```python
from build123d import *

# Parameters (mm, degrees)
F0_W           = 40
F0_H           = 40
F0_R           = 0.75
F0_W_2         = 13
F0_H_2         = 14
F1_DEPTH       = 10
F3_DEPTH       = 7
F5_DEPTH       = 7
F6_W           = 1
F6_H           = 10
F7_DEPTH       = 3
F9_W           = 40
F9_H           = 40
F9_W_2         = 13
F9_H_2         = 14
F10_DEPTH      = 5
F8_W           = 16.9138771733
F8_H           = 9.9888166223
F11_DEPTH      = 5
F13_W          = 3
F13_H          = 1.8063458446
F13_H_2        = 1.6774383839
F14_DEPTH      = 7
F15_W          = 50
F15_H          = 50
F15_W_2        = 40
F15_H_2        = 40
F16_DEPTH      = 10
F16_DEPTH_BACK = 5
F8_W_2         = 1
F8_W_3         = 4.5249774149
F8_W_4         = 11.3888997585
F18_DEPTH      = 5
F17_R          = 2.5
F19_DEPTH      = 15
F20_W          = 1
F20_H          = 18
F20_W_2        = 1.1054268107
F20_H_2        = 4.0429783403
F20_H_3        = 1.6282203142
F20_W_3        = 3.4427661449
F20_H_4        = 4.0144510567
F21_DEPTH      = 7
F22_W          = 1.9634229802
F22_H          = 1
F23_DEPTH      = 3


with BuildPart() as f1:
    # F0 (on Top) → F1 (new body)
    with BuildSketch(Plane.XY):
        with Locations((3.7967593362, -3.7976530202)):
            Rectangle(F0_W, F0_H)
        with Locations((-5.9532406638, -3.7976530202)):
            Circle(F0_R, mode=Mode.SUBTRACT)
        with Locations((3.7967593362, -3.7976530202)):
            Rectangle(F0_W_2, F0_H_2, mode=Mode.SUBTRACT)
    extrude(amount=F1_DEPTH)

    # F2 (on face) → F3 (cut)
    with BuildSketch(Plane.XY.offset(10)):
        Polygon((10.2967593362, -10.7976530202), (-2.7032406638, -10.7976530202), (19.3193775079, -11.9658830875), (19.2741411646, 5.0340567263), (-2.7032406638, 3.2023469798), (10.2967593362, 3.2023469798), (10.2967593362, -1.4381406363), (10.2967593362, -5.3588831797), align=None)
    extrude(amount=-F3_DEPTH, mode=Mode.SUBTRACT)

    # F4 (on face) → F5 (join)
    with BuildSketch(Plane.XY.offset(3)):
        Polygon((10.2967593362, -3.7976530202), (10.2967593362, -8.2976530202), (14.2967593362, -8.2976530202), (14.2967593362, 0.7023469798), (10.2967593362, 0.7023469798), align=None)
    extrude(amount=F5_DEPTH)

    # F6 (on face) → F7 (cut)
    with BuildSketch(Plane.XY.offset(3)):
        with Locations((18.7717819214, -3.4659131806)):
            Rectangle(F6_W, F6_H)
    extrude(amount=-F7_DEPTH, mode=Mode.SUBTRACT)

    # F9 (on face) → F10 (join)
    with BuildSketch(Plane(origin=(0, 0, 0), x_dir=(1, 0, 0), z_dir=(0, 0, -1))):
        with Locations((3.7967593362, 3.7976530202)):
            Rectangle(F9_W, F9_H)
        with Locations((3.7967593362, 3.7976530202)):
            Rectangle(F9_W_2, F9_H_2, mode=Mode.SUBTRACT)
    extrude(amount=F10_DEPTH)

    # F8 (on face) → F11 (cut)
    with BuildSketch(Plane(origin=(0, 0, 0), x_dir=(1, 0, 0), z_dir=(0, 0, -1))):
        with Locations((26.728720508, 3.4603214917)):
            Rectangle(F8_W, F8_H)
    extrude(amount=-F11_DEPTH, mode=Mode.SUBTRACT)

    # F13 (on face) → F14 (cut)
    with BuildSketch(Plane.XY.offset(10)):
        Polygon((19.5070204958, -12.4706726056), (19.5070204958, 5.5293273944), (15.5070204958, 5.5293273944), (15.5070204958, 3.7229815498), (15.5070204958, -10.7932342216), (15.5070204958, -12.4706726056), align=None)
        with Locations((14.0070204958, 4.6261544721)):
            Rectangle(F13_W, F13_H)
        with Locations((14.0070204958, -11.6319534136)):
            Rectangle(F13_W, F13_H_2)
    extrude(amount=-F14_DEPTH, mode=Mode.SUBTRACT)

    # F15 (on Top) → F16 (join, two sides)
    with BuildSketch(Plane.XY) as f16_sk:
        with Locations((3.7967593362, -3.7976530202)):
            Rectangle(F15_W, F15_H)
        with Locations((3.7967593362, -3.7976530202)):
            Rectangle(F15_W_2, F15_H_2, mode=Mode.SUBTRACT)
    extrude(amount=F16_DEPTH)
    extrude(f16_sk.sketch, amount=-F16_DEPTH_BACK)

    # F8 (on face) → F18 (cut)
    with BuildSketch(Plane(origin=(0, 0, 0), x_dir=(1, 0, 0), z_dir=(0, 0, -1))):
        with Locations((18.7717819214, 3.4603214917)):
            Rectangle(F8_W_2, F8_H)
        with Locations((21.5342706288, 3.4603214917)):
            Rectangle(F8_W_3, F8_H)
        with Locations((29.4912092155, 3.4603214917)):
            Rectangle(F8_W_4, F8_H)
    extrude(amount=-F18_DEPTH, mode=Mode.SUBTRACT)

    # F17 (on face) → F19 (cut)
    with BuildSketch(Plane.XY.offset(10)):
        with Locations((-16.2032406638, -23.7976530202)):
            Circle(F17_R)
        with Locations((-16.2032406638, 16.2023469798)):
            Circle(F17_R)
        with Locations((23.7967593362, -23.7976530202)):
            Circle(F17_R)
        with Locations((23.7967593362, 16.2023469798)):
            Circle(F17_R)
    extrude(amount=-F19_DEPTH, mode=Mode.SUBTRACT)

    # F20 (on face) → F21 (cut)
    with BuildSketch(Plane.XY.offset(10)):
        with Locations((20.0070204958, -3.4706726056)):
            Rectangle(F20_W, F20_H)
        with Locations((14.2178074457, -1.1141116556)):
            Rectangle(F20_W_2, F20_H_2)
        with Locations((14.2178074457, -3.9497109829)):
            Rectangle(F20_W_2, F20_H_3)
        with Locations((11.9437109679, -3.9497109829)):
            Rectangle(F20_W_3, F20_H_3)
        with Locations((14.2178074457, -6.7710466683)):
            Rectangle(F20_W_2, F20_H_4)
    extrude(amount=-F21_DEPTH, mode=Mode.SUBTRACT)

    # F22 (on face) → F23 (cut)
    with BuildSketch(Plane.XY.offset(10)):
        with Locations((-2.7032406638, -3.7976530202)):
            Rectangle(F22_W, F22_H)
    extrude(amount=-F23_DEPTH, mode=Mode.SUBTRACT)


solid = f1.part
```
Geometry check sheet. Reference: the model listing, model coordinates, mm. A direction names the side the tool comes from. Give positions to 0.01 mm unless a question says otherwise; leave off trailing zeros. Order: outer loops, then holes, each group sorted by start corner. A loop starts at its lowest first (then second) coordinate and runs counter-clockwise, first axis right, second up. Notation, with made-up numbers: (4, 0.5) -> (35, 0.5) arc R17 cw to (35, 22.5) -> close; hole circle Ø4 at (-39, 57). An arc over 180 degrees is marked (long way). Write each question's results on one line, items separated by ' | '. Start each with the question number.
(1) Access from +Z, -Z, +X, -X, +Y, -Y to the whole of each face (thin tool, end or side, straight path). Record for faces 5 (the face through (12, -4.764, 7)), 6 (the face through (3, 8, -5)), 7 (the face through (10.297, -4, 1)), 8 (the face through (28.797, -4, -1)), 9 (the face through (25, -4, 5)).
(2) Scan lines: line 1 (Y direction, x = -16, z = 1.5); line 2 (Y direction, x = -6.5, z = 0.5); line 3 (X direction, y = 15.5, z = 2). Record each from-to range of solid material in increasing order.
(3) Sectioned sample at C-C (z = -1). Enter the section's corners in (x, y).
(4) Mould release check, pull along X, two halves, no side actions. Record for faces 1 (the face through (16, -12.471, 7)), 2 (the face through (3, -28.798, 3)), 3 (the face through (21.8, 14.7, 2.6)), 4 (the face through (-21.203, -4, 3)): pulls with the +X half, pulls with the -X half, needs draft (parallel to the pull), parting line crosses it, or undercut.
(5) Sectioned sample at A-A (z = 6.25). Give the number of separate pieces and of enclosed holes in the cut face, plus the area to 3 significant figures.
(6) Sectioned sample at B-B (x = 25). Enter the section's corners in (y, z).
Answer below:
1) face 5: +Z | face 6: -Z, +X, -X, +Y, -Y | face 7: +Z, -Z | face 8: +Z, -Z, +X, +Y, -Y | face 9: +X
2) line 1: -28.8 to -26.29, -21.31 to 13.71, 18.69 to 21.2 | line 2: -28.8 to -4.31, -3.28 to 21.2 | line 3: -21.2 to -18.6, -13.8 to 21.4, 26.2 to 28.8
3) outline: (-21.2, -28.8) -> (28.8, -28.8) -> (28.8, 21.2) -> (-21.2, 21.2) -> close; hole circle Ø5 at (-16.2, -23.8); hole circle Ø5 at (-16.2, 16.2); hole (-2.7, -10.8) -> (10.3, -10.8) -> (10.3, 3.2) -> (-2.7, 3.2) -> close; hole circle Ø5 at (23.8, -23.8); hole circle Ø5 at (23.8, 16.2)
4) face 1: undercut | face 2: needs draft | face 3: undercut | face 4: pulls with the -X half
5) separate pieces: 3 | enclosed holes: 6 | area: 2,070 mm2
6) outline: (-28.8, -5) -> (-25.99, -5) -> (-25.99, 10) -> (-28.8, 10) -> close; (-21.61, -5) -> (14.01, -5) -> (14.01, 10) -> (-21.61, 10) -> close; (18.39, -5) -> (21.2, -5) -> (21.2, 10) -> (18.39, 10) -> close; hole (-8.45, 0) -> (1.53, 0) -> (1.53, 5) -> (-8.45, 5) -> close
